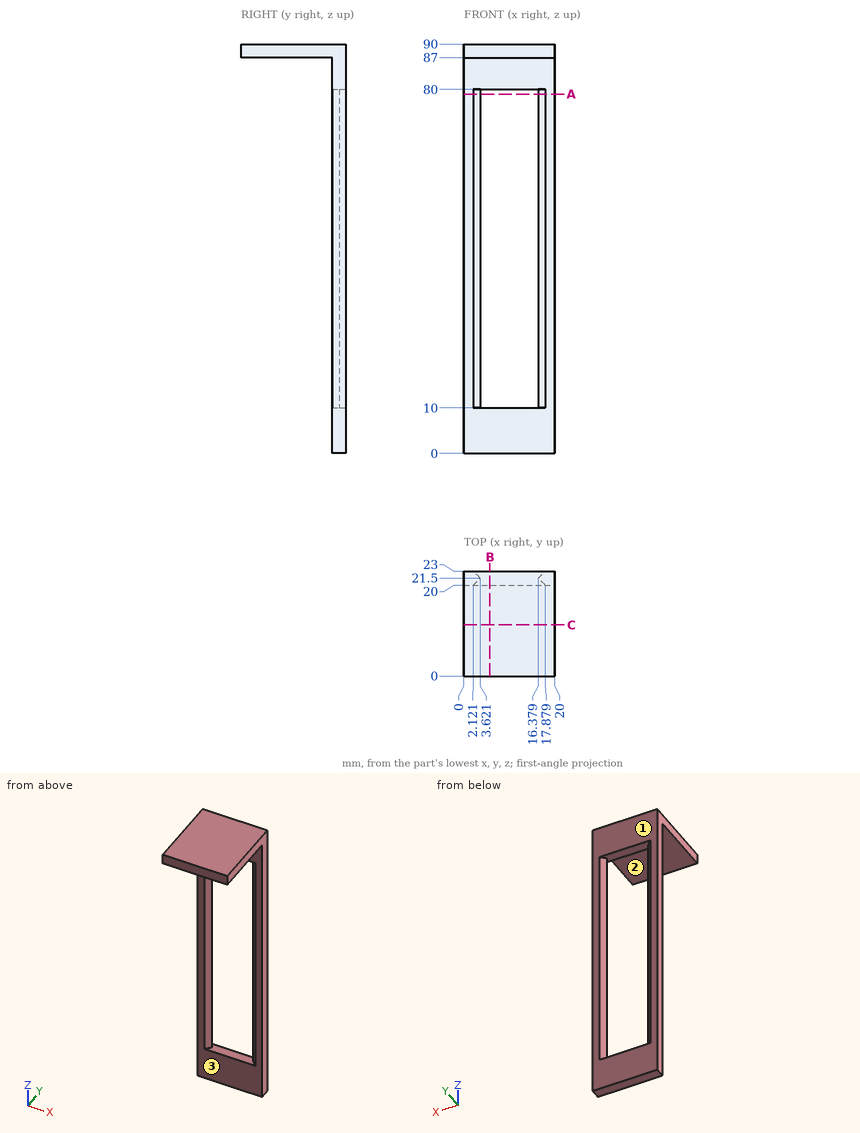
Here's the drawing with two shaded views (mm, measured from the low corner). I have some questions. Coordinates: 2 decimals unless noted, no trailing zeros. Write each loop counter-clockwise with the first axis right and the second up, starting at its lowest first coordinate (ties: lowest second). Pieces come first, ordered by that corner, then holes. Notation, with made-up numbers: M 83,15 L 121,15 A29 cw 121,49 Z; hole C 44.25,25 d10. An arc over 180 degrees is marked long. Answer as CSV lines item,"result".
Item 1: Please list where these lines run through material, in increasing order: line 1 along Z through (x, y) = (3.25, 20.75); line 2 along Z through (x, y) = (6.5, 15.5); line 3 along Y through (x, z) = (8.5, 80.5).
Geometry results:
line 1,"z = 0 to 10, 80 to 90"
line 2,"z = 87 to 90"
line 3,"y = 20 to 23"
Item 2: I'm going to push flat-ended pins straight in: P1, Ø8, axis at x = 11.5, z = 74, coming from the +Y side; P2, Ø2.5, axis at x = 9.5, y = 21.5, coming from the -Z side; P3, Ø10, axis at x = 12, z = 55, coming from the -Y side; P4, Ø3, axis at x = 5, z = 17.5, coming from the -Y side. Where does each tip first touch, or does it pass through?
Geometry results:
P1,"passes through"
P2,"stops at z = 0"
P3,"stops at y = 20.88"
P4,"stops at y = 21.38"
Item 3: Imagine slicing it at A-A on z = 79. List the corners of the cut face in (x, y) for me.
Geometry results:
outline,"M 0,20 L 2.12,20 L 3.62,21.5 L 2.12,23 L 0,23 Z; M 16.38,21.5 L 17.88,20 L 20,20 L 20,23 L 17.88,23 Z"
Item 4: We'd pull the mould along Y, two halves only. Please class the marked faces 1, 2 and 3: +Y half, -Y half, draft (parallel to the pull), parting line (faces both ways), or undercut.
Geometry results:
face 1,"+Y half"
face 2,"draft"
face 3,"-Y half"
Item 5: Imagine slicing it at C-C on y = 11.25. List the corners of the cut face in (x, z) for me, plus the area to 3 significant figures.
Geometry results:
outline,"M 0,87 L 20,87 L 20,90 L 0,90 Z"
area,"60.0 mm2"
Item 6: Imagine slicing it at B-B on x = 5.75. List the corners of the cut face in (y, z) for me.
Geometry results:
outline,"M 0,87 L 20,87 L 20,80 L 23,80 L 23,90 L 0,90 Z; M 20,0 L 23,0 L 23,10 L 20,10 Z"
